```python
from build123d import *

# Parameters (mm, degrees)
SKETCH1_W                 = 14.7
SKETCH1_H                 = 14.7
BOSS_EXTRUDE1_DEPTH       = 76.2
SKETCH6_R                 = 3.175
CUT_EXTRUDE4_DEPTH        = 78.952244997
CHAMFER5_SIZE             = 1
CHAMFER6_SIZE             = 2.54
SKETCH4_W                 = 35.56
SKETCH4_H                 = 20.32
BOSS_EXTRUDE2_DEPTH       = 30.48
SKETCH5_R                 = 3.175
TRAYSUPPORTMOUNTING_DEPTH = 106.430644976
CHAMFER4_SIZE             = 1
CUT_EXTRUDE5_DEPTH        = 27.94
FILLET1_R                 = 6.35
SKETCH8_R                 = 1.4
CUT_EXTRUDE6_DEPTH        = 103.768035887


with BuildPart() as part:
    # Sketch1 → Boss-Extrude1 (new body)
    with BuildSketch(Plane(origin=(0, 0, 0), x_dir=(1, 0, 0), z_dir=(0, 1, 0))):
        Rectangle(SKETCH1_W, SKETCH1_H)
    extrude(amount=BOSS_EXTRUDE1_DEPTH)

    # Sketch6 → Cut-Extrude4 (cut, through all)
    with BuildSketch(Plane(origin=(7.35, 0, 0), x_dir=(0, 0, -1), z_dir=(1, 0, 0))):
        with Locations((0, 65.405)):
            Circle(SKETCH6_R)
        with Locations((0, 51.435)):
            Circle(SKETCH6_R)
        with Locations((0, 37.465)):
            Circle(SKETCH6_R)
        with Locations((0, 23.495)):
            Circle(SKETCH6_R)
        with Locations((0, 9.525)):
            Circle(SKETCH6_R)
    extrude(amount=-CUT_EXTRUDE4_DEPTH, mode=Mode.SUBTRACT)

    # Chamfer5
    chamfer5_edges = [part.edges().sort_by_distance(p)[0] for p in [
        (-7.35, 65.405, 3.175),
        (7.35, 65.405, 3.175),
        (-7.35, 51.435, 3.175),
        (7.35, 51.435, 3.175),
        (-7.35, 37.465, 3.175),
        (7.35, 37.465, 3.175),
        (-7.35, 23.495, 3.175),
        (7.35, 23.495, 3.175),
    ]]
    chamfer(chamfer5_edges, length=CHAMFER5_SIZE)

    # Chamfer6
    chamfer6_edges = [part.edges().sort_by_distance(p)[0] for p in [
        (0, 0, -7.35),
        (7.35, 0, 0),
        (0, 0, 7.35),
        (-7.35, 0, 0),
    ]]
    chamfer(chamfer6_edges, length=CHAMFER6_SIZE)

    # Sketch4 → Boss-Extrude2 (add)
    with BuildSketch(Plane.XY.offset(7.35)):
        with Locations((0, 86.36)):
            Rectangle(SKETCH4_W, SKETCH4_H)
    extrude(amount=-BOSS_EXTRUDE2_DEPTH)

    # Sketch5 → TraySupportMounting (cut, through all)
    with BuildSketch(Plane(origin=(17.78, 0, 0), x_dir=(0, 0, -1), z_dir=(1, 0, 0))):
        with Locations((9.16, 88.9)):
            Circle(SKETCH5_R)
        with Locations((-2.27, 88.9)):
            Circle(SKETCH5_R)
    extrude(amount=-TRAYSUPPORTMOUNTING_DEPTH, mode=Mode.SUBTRACT)

    # Chamfer4
    chamfer4_edges = [part.edges().sort_by_distance(p)[0] for p in [
        (-17.78, 88.9, -5.985),
        (17.78, 88.9, -5.985),
        (-17.78, 88.9, 5.445),
        (17.78, 88.9, 5.445),
    ]]
    chamfer(chamfer4_edges, length=CHAMFER4_SIZE)

    # Sketch7 → Cut-Extrude5 (cut)
    with BuildSketch(Plane(origin=(0, 0, -23.13), x_dir=(-1, 0, 0), z_dir=(0, 0, -1))):
        Polygon((-6.35, 96.52), (-7.830526815, 93.345), (7.830526815, 93.345), (6.35, 96.52), align=None)
    extrude(amount=-CUT_EXTRUDE5_DEPTH, mode=Mode.SUBTRACT)

    # Fillet1
    fillet1_edges = [part.edges().sort_by_distance(p)[0] for p in [
        (-17.78, 86.36, -23.13),
        (17.78, 86.36, -23.13),
    ]]
    fillet(fillet1_edges, radius=FILLET1_R)

    # Sketch8 → Cut-Extrude6 (cut, through all)
    with BuildSketch(Plane.XY.offset(7.35)):
        with Locations((0, 93.98)):
            Circle(SKETCH8_R)
    extrude(amount=-CUT_EXTRUDE6_DEPTH, mode=Mode.SUBTRACT)


solid = part.part
```
Source: CAD feature listing. Evaluate the final solid. Frame: model axes, mm. A direction names the side the tool comes from. Round coordinates to 2 decimals unless told otherwise and drop trailing zeros. Write each loop counter-clockwise with the first axis right and the second up, starting at its lowest first coordinate (ties: lowest second). Pieces come first, ordered by that corner, then holes. Notation, with made-up numbers: M -1,80 L 11,80 A22 ccw 11,90 Z; hole C 22,-20 d10. An arc over 180 degrees is marked long. Use CSV: the item, a comma, the result in double quotes. Start each with the question number.
Q1. First-contact query: P1, Ø7.5, axis at y = 23.495, z = 0, coming from the +X side (3 decimals); P2, Ø5.5, axis at y = 9.525, z = 0, coming from the +X side (1 decimal); P3, Ø1, axis at y = 40.5, z = -5.5, coming from the +X side; P4, Ø12, axis at x = 0.5, y = 56, coming from the -Z side. Flat tips, straight axial feed; report the tip coordinate or a pass-through.
Q2. Access query for faces 4 (the face through (0, 39, -7.35)), 5 (the face through (5, 93.345, -9)), 6 (the face through (7.35, 39, 5)), 7 (the face through (0.089, 26.643, 0.413)). Directions: +Z, -Z, +X, -X, +Y, -Y. A direction counts if a zero-diameter tool reaches every point of the face in a straight line with its end or side. Return the directions, or none.
Q3. Cut plane C-C on z = -21. Output: boundary loops of the cut face in (x, y) (3 decimals), plus the area to 3 significant figures.
Q4. Pull-direction query (X, two-part tool) for faces 1 (the face through (-0.303, 92.613, -4.29)), 2 (the face through (0.23, 85.8, 2.96)), 3 (the face through (-6.06, 1.25, 0.1)); classes: +X half, -X half, draft (parallel to the pull), parting line (faces both ways), or undercut.
Q5. Cut plane A-A on y = 88.9. Output: boundary loops of the cut face in (x, z) (3 decimals), plus the area to 3 significant figures.
Q6. Line query: line 1 (Y direction, x = 4, z = -1.5) (3 decimals); line 2 (Z direction, x = -4, y = 88); line 3 (Y direction, x = -5, z = -14) (3 decimals). Output: solid intervals per line, ascending. Write a range as from..to.
Q7. Cut plane B-B on x = 0. Count the separate pieces of the cut face and the enclosed holes in it, plus the area to 3 significant figures.
Results found:
1,P1,"x = 6.925"
1,P2,"through"
1,P3,"x = 7.35"
1,P4,"z = -7.35"
2,face 4,"-Z, +X, -X, -Y"
2,face 5,"-Z"
2,face 6,"+Z, -Z, +X, -Y"
2,face 7,"+X, -X"
3,outline,"M -16.175,76.2 L 16.175,76.2 L 16.175,96.52 L 6.35,96.52 L 7.831,93.345 L 1.248,93.345 A1.4 cw -1.248,93.345 L -7.831,93.345 L -6.35,96.52 L -16.175,96.52 Z"
3,area,"611 mm^2"
4,face 1,"undercut"
4,face 2,"draft"
4,face 3,"-X half"
5,outline,"M -17.78,-16.78 A6.35 ccw -11.43,-23.13 L 11.43,-23.13 A6.35 ccw 17.78,-16.78 L 17.78,-13.335 L 16.78,-12.335 L -16.78,-12.335 L -17.78,-13.335 Z; M -17.78,-4.985 L -16.78,-5.985 L 16.78,-5.985 L 17.78,-4.985 L 17.78,-1.905 L 16.78,-0.905 L -16.78,-0.905 L -17.78,-1.905 Z; M -17.78,6.445 L -16.78,5.445 L 16.78,5.445 L 17.78,6.445 L 17.78,7.35 L -17.78,7.35 Z"
5,area,"611 mm^2"
6,line 1,"0..6.727, 12.323..20.697, 26.293..34.667, 40.263..48.637, 54.233..62.607, 68.203..93.345"
6,line 2,"-23.13..-12.2, -6.12..-0.77, 5.31..7.35"
6,line 3,"76.2..93.345"
7,separate pieces,"2"
7,enclosed holes,"7"
7,area,"1,390 mm^2"
